Could you check a few things on this model? Use its own coordinates, in mm. A direction names the side the tool comes from. Round coordinates to 2 decimals unless told otherwise and drop trailing zeros. Write each loop counter-clockwise with the first axis right and the second up, starting at its lowest first coordinate (ties: lowest second). Pieces come first, ordered by that corner, then holes. Notation, with made-up numbers: (-34, 23) - (-30, 23) arc R10 cw to (-30, 35) - close; hole circle Ø3 at (77.25, 64). An arc over 180 degrees is marked (long way). Write each question's results on one line, items separated by ' | '. Start each with the question number.
(1) For P1, Ø1.5, axis at x = 5, y = 5, coming from the -Z side; P2, Ø3, axis at y = 0, z = -3, coming from the +X side; P3, Ø2.5, axis at x = -1, z = -1.5, coming from the +Y side, each with a flat end and sliding along its axis, tell me the tip position at first contact or that it passes through.
(2) Thinking about a two-plate mould opening in Z: for faces 1 (the cylindrical face through (-1.172, -6.24, -8.923)), 2 (the cylindrical face through (-0.59, 5.52, -4.46)), 3 (the cylindrical face through (-3, 0, 0)), 4 (the flat face through (4, 7, 4)), which applies, +Z half, -Z half, draft (parallel to the pull), parting line (faces both ways), or undercut?
(3) Imagine slicing it at C-C on y = 4.5. Write out the boundary of the cut face in (x, z).
(4) Imagine slicing it at B-B on z = 0. Write out the boundary of the cut face in (x, y).
(5) On a 3-axis mill with a long thin cutter (end or side, diameter ignored), from which of +Z, -Z, +X, -X, +Y, -Y can I reach the whole of each face in a straight line? I mean faces 5 (the cylindrical face through (-0.59, -5.48, -4.46)), 6 (the cylindrical face through (-1.172, 6.24, -8.923)), 7 (the flat face through (2, -5.5, 6)), 8 (the flat face through (4, -7, 4)), 9 (the flat face through (1, 4, 3)). Say none if no direction works.
(6) Imagine slicing it at D-D on z = -3.75. Write out the boundary of the cut face in (x, y).
(7) Imagine slicing it at A-A on x = 0. Write out the boundary of the cut face in (y, z).
(8) Please list where these lines run through material, in increasing order: line 1 (X direction, y = -6.1, z = 0); line 2 (Z direction, x = 0, y = -0.5). Write a range as [from, to].
```python
from build123d import *

# Parameters (mm, degrees)
SKETCH1_R           = 6
SKETCH1_R_2         = 4.5
BOSS_EXTRUDE1_DEPTH = 5.5
SKETCH2_R           = 9
SKETCH2_R_2         = 4.5
BOSS_EXTRUDE2_DEPTH = 1.5
SKETCH3_R           = 4.5
SKETCH3_R_2         = 3
BOSS_EXTRUDE3_DEPTH = 4


with BuildPart() as part:
    # Sketch1 → Boss-Extrude1 (new body, symmetric)
    with BuildSketch(Plane(origin=(0, 0, 0), x_dir=(1, 0, 0), z_dir=(0, 1, 0))):
        Circle(SKETCH1_R)
        Circle(SKETCH1_R_2, mode=Mode.SUBTRACT)
    extrude(amount=BOSS_EXTRUDE1_DEPTH, both=True)

    # Sketch2 → Boss-Extrude2 (add)
    with BuildSketch(Plane(origin=(0, 5.5, 0), x_dir=(1, 0, 0), z_dir=(0, 1, 0))):
        Circle(SKETCH2_R)
        Circle(SKETCH2_R_2, mode=Mode.SUBTRACT)
    boss_extrude2 = extrude(amount=BOSS_EXTRUDE2_DEPTH)

    # Mirror1: Boss-Extrude2 across plane
    add(boss_extrude2.mirror(Plane.ZX))

    # Sketch3 → Boss-Extrude3 (add, symmetric)
    with BuildSketch(Plane(origin=(0, 0, 0), x_dir=(1, 0, 0), z_dir=(0, 1, 0))):
        Circle(SKETCH3_R)
        Circle(SKETCH3_R_2, mode=Mode.SUBTRACT)
    extrude(amount=BOSS_EXTRUDE3_DEPTH, both=True)


solid = part.part
```
Response:
1) P1: z = -7.83 | P2: x = 5.81 | P3: y = 4
2) face 1: parting line | face 2: undercut | face 3: undercut | face 4: draft
3) outline: circle Ø12 at (0, 0); hole circle Ø9 at (0, 0)
4) outline: (-9, -7) - (-4.5, -7) - (-4.5, -4) - (-3, -4) - (-3, 4) - (-4.5, 4) - (-4.5, 7) - (-9, 7) - (-9, 5.5) - (-6, 5.5) - (-6, -5.5) - (-9, -5.5) - close; (3, -4) - (4.5, -4) - (4.5, -7) - (9, -7) - (9, -5.5) - (6, -5.5) - (6, 5.5) - (9, 5.5) - (9, 7) - (4.5, 7) - (4.5, 4) - (3, 4) - close
5) face 5: -Y | face 6: +Y, -Y | face 7: none | face 8: +Z, -Z, +X, -X, -Y | face 9: +Y
6) outline: (-8.18, -7) - (-2.49, -7) - (-2.49, -4) - (2.49, -4) - (2.49, -7) - (8.18, -7) - (8.18, -5.5) - (4.68, -5.5) - (4.68, 5.5) - (8.18, 5.5) - (8.18, 7) - (2.49, 7) - (2.49, 4) - (-2.49, 4) - (-2.49, 7) - (-8.18, 7) - (-8.18, 5.5) - (-4.68, 5.5) - (-4.68, -5.5) - (-8.18, -5.5) - close
7) outline: (-7, -9) - (-5.5, -9) - (-5.5, -6) - (5.5, -6) - (5.5, -9) - (7, -9) - (7, -4.5) - (4, -4.5) - (4, -3) - (-4, -3) - (-4, -4.5) - (-7, -4.5) - close; (-7, 4.5) - (-4, 4.5) - (-4, 3) - (4, 3) - (4, 4.5) - (7, 4.5) - (7, 9) - (5.5, 9) - (5.5, 6) - (-5.5, 6) - (-5.5, 9) - (-7, 9) - close
8) line 1: [-9, -4.5], [4.5, 9] | line 2: [-6, -3], [3, 6]
